Input: dimensioned drawing with shaded views. Units: mm. Origin: part minimum x, y, z. A direction names the side the tool comes from. Give positions to 0.01 mm unless a question says otherwise; leave off trailing zeros. Write each loop counter-clockwise with the first axis right and the second up, starting at its lowest first coordinate (ties: lowest second). Pieces come first, ordered by that corner, then holes. Notation, with made-up numbers: (45.5, 26) -> (58.5, 26) arc R30 cw to (58.5, 64) -> close; hole circle Ø7 at (-35, -3). An arc over 180 degrees is marked (long way). Answer as a JSON object with one key per item and string values.
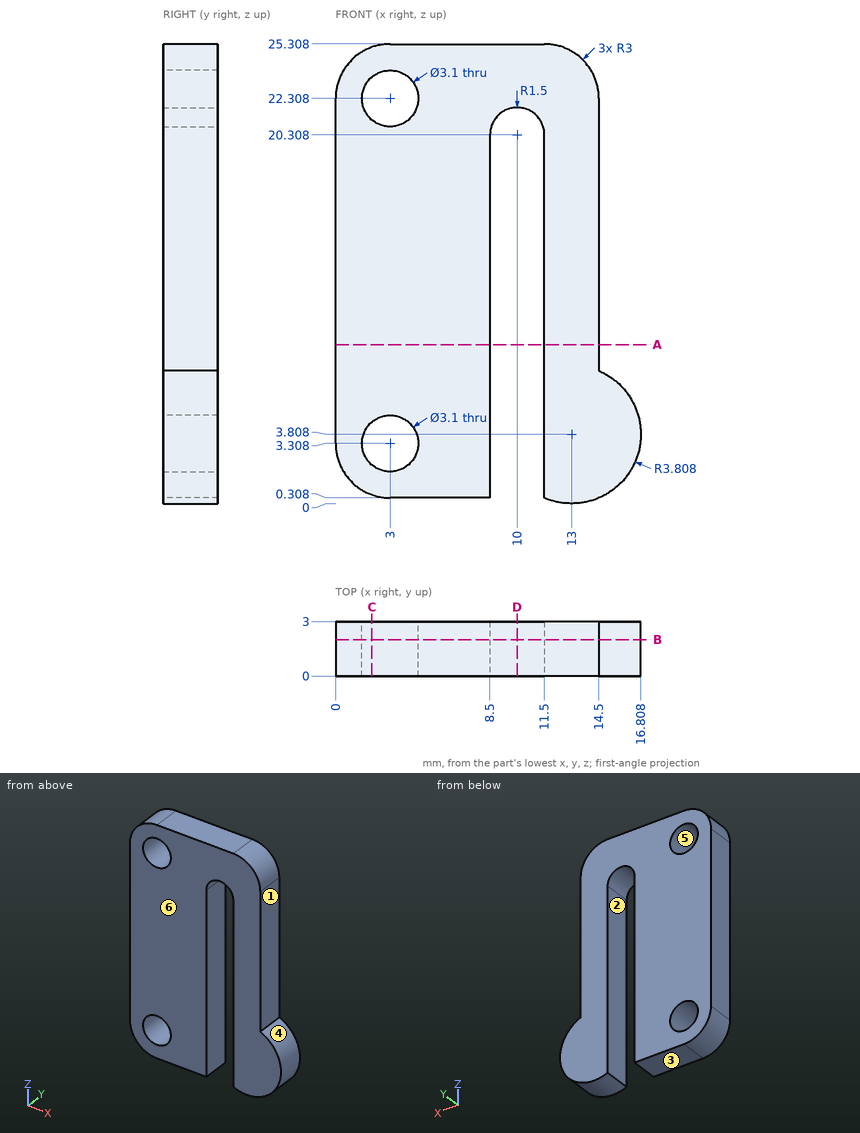
Q1. Material intervals for L1, parallel to X at y = 0.7, z = 12; L2, parallel to X at y = 0.35, z = 4; L3, parallel to X at y = 0.2, z = 21, sorted ascending. Write a range as from..to.
Values:
{"L1": "0..8.5, 11.5..14.5", "L2": "0..1.61, 4.39..8.5, 11.5..16.8", "L3": "0..2.17, 3.83..8.67, 11.33..14.5"}
Q2. Cut plane A-A (z = 8.75). Return the cut outline in (x, y), and give its area (3 significant figures).
Values:
{"outline": "(0, 0) -> (8.5, 0) -> (8.5, 3) -> (0, 3) -> close; (11.5, 0) -> (14.5, 0) -> (14.5, 3) -> (11.5, 3) -> close", "area": "34.5 mm²"}
Q3. Set-up query: the marked faces 1, 2 and 3. Return all of +Z, -Z, +X, -X, +Y, -Y with unobstructed straight access to the full face (end or side cutting, diameter ignored); none if empty.
Values:
{"face 1": "+Z, +X, +Y, -Y", "face 2": "-Z, +Y, -Y", "face 3": "-Z, -X, +Y, -Y"}
Q4. Mould query, pull axis Z, two halves, no side actions, for the marked faces 4, 5 and 6. Classes: pulls with the +Z half, pulls with the -Z half, needs draft (parallel to the pull), parting line crosses it, or undercut.
Values:
{"face 4": "parting line crosses it", "face 5": "undercut", "face 6": "needs draft"}
Q5. Cut plane C-C (x = 2). Return the cut outline in (y, z).
Values:
{"outline": "(0, 0.48) -> (3, 0.48) -> (3, 2.12) -> (0, 2.12) -> close; (0, 4.49) -> (3, 4.49) -> (3, 21.12) -> (0, 21.12) -> close; (0, 23.49) -> (3, 23.49) -> (3, 25.14) -> (0, 25.14) -> close"}
Q6. First-contact query: P1, Ø0.9, axis at y = 2, z = 13, coming from the +X side. Flat tip, straight axial feed; report the tip coordinate or a pass-through.
Values:
{"P1": "x = 14.5"}
Q7. Cut plane D-D (x = 10). Return the cut outline in (y, z).
Values:
{"outline": "(0, 21.81) -> (3, 21.81) -> (3, 25.31) -> (0, 25.31) -> close"}
Q8. Cut plane B-B (y = 2). Return the cut outline in (x, z), and give its area (3 significant figures).
Values:
{"outline": "(0, 3.31) arc R3 ccw to (3, 0.31) -> (8.5, 0.31) -> (8.5, 20.31) arc R1.5 cw to (11.5, 20.31) -> (11.5, 0.31) arc R3.81 ccw to (14.5, 7.31) -> (14.5, 22.31) arc R3 ccw to (11.5, 25.31) -> (3, 25.31) arc R3 ccw to (0, 22.31) -> close; hole circle Ø3.1 at (3, 3.31); hole circle Ø3.1 at (3, 22.31)", "area": "290 mm²"}
